Input: part model. Units: mm. Frame: model coordinates. Face numbers are marked on the shaded views. A direction names the side the tool comes from. Give positions to 0.01 mm unless a question says otherwise; leave off trailing zeros. Order: outer loops, then holes, each group sorted by start corner. A loop starts at its lowest first (then second) coordinate and runs counter-clockwise, first axis right, second up. Notation, with made-up numbers: M 50.5,-13 L 107.5,-13 A19 cw 107.5,8 Z; hole C 61.5,66 d2. An arc over 180 degrees is marked long. Use a Markdown table: item, result.
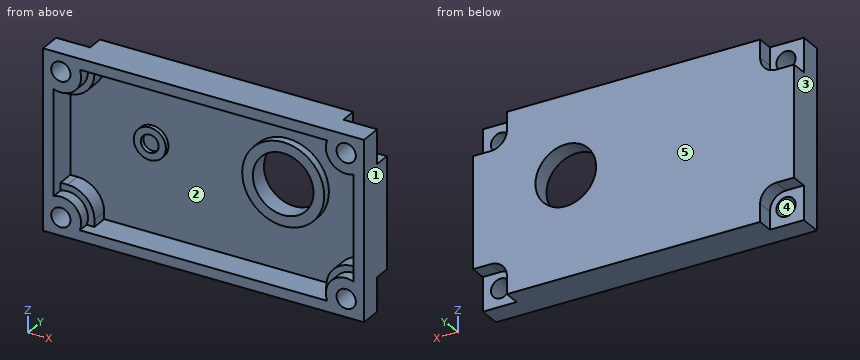
from build123d import *

# Parameters (mm, degrees)
SKETCH_1_W            = 45
SKETCH_1_H            = 25
EXTRUDE_1_DEPTH       = 5.4
SKETCH_2_R            = 1.35
CUT_EXTRUDE_1_DEPTH   = 27.299429652
CUT_EXTRUDE_2_DEPTH   = 2.3
MIRROR_2_COPY_1_DEPTH = 2.3
SHELL_1_DEPTH         = 3.9
SHELL_1_2_DEPTH       = 1.6
SKETCH_4_R            = 4.25
CUT_EXTRUDE_3_DEPTH   = 27.299429652
SKETCH_6_R            = 5.75
SKETCH_6_R_2          = 4.25
EXTRUDE_3_DEPTH       = 1.1
SKETCH_7_R            = 2.25
SKETCH_7_R_2          = 1.25
EXTRUDE_4_DEPTH       = 0.6


# Read off the part's stored shape, not the designer's step: 薄殼1
with BuildPart() as part:
    # 草圖1 → 填料-伸長1 (new body)
    with BuildSketch(Plane(origin=(0, 0, 0), x_dir=(1, 0, 0), z_dir=(0, 1, 0))):
        Rectangle(SKETCH_1_W, SKETCH_1_H)
    extrude(amount=EXTRUDE_1_DEPTH)

    # 草圖2 → 除料-伸長1 (cut, through all)
    with BuildSketch(Plane(origin=(0, 5.4, 0), x_dir=(1, 0, 0), z_dir=(0, 1, 0))):
        with Locations(Location((-20, 10, 0), (0, 0, 270))):
            Circle(SKETCH_2_R)
        with Locations(Location((-20, -10, 0), (0, 0, 270))):
            Circle(SKETCH_2_R)
        with Locations(Location((20, -10, 0), (0, 0, 270))):
            Circle(SKETCH_2_R)
        with Locations(Location((20, 10, 0), (0, 0, 270))):
            Circle(SKETCH_2_R)
    extrude(amount=-CUT_EXTRUDE_1_DEPTH, mode=Mode.SUBTRACT)

    # 草圖3 → 除料-伸長2 (cut)
    with BuildSketch(Plane(origin=(0, 5.4, 0), x_dir=(1, 0, 0), z_dir=(0, 1, 0))):
        with BuildLine():
            Line((-20, -7.75), (-22.5, -7.75))
            Line((-22.5, -7.75), (-22.5, -12.5))
            Line((-22.5, -12.5), (-17.75, -12.5))
            Line((-17.75, -12.5), (-17.75, -10))
            ThreePointArc((-17.75, -10), (-18.409009742, -8.409009742), (-20, -7.75))
        make_face()
    cut_extrude_2 = extrude(amount=-CUT_EXTRUDE_2_DEPTH, mode=Mode.SUBTRACT)

    # 鏡射1: 除料-伸長2 across plane
    add(cut_extrude_2.mirror(Plane.XY), mode=Mode.SUBTRACT)

    # 鏡射2: 除料-伸長2 across plane
    add(cut_extrude_2.mirror(Plane(origin=(0, 0, 0), x_dir=(0, 0, 1), z_dir=(1, 0, 0))), mode=Mode.SUBTRACT)

    # 鏡射2 copy 1 sketch → 鏡射2 copy 1 (cut)
    with BuildSketch(Plane(origin=(0, 5.4, 0), x_dir=(-1, 0, 0), z_dir=(0, 1, 0))):
        with BuildLine():
            Line((-20, -7.75), (-22.5, -7.75))
            Line((-22.5, -7.75), (-22.5, -12.5))
            Line((-22.5, -12.5), (-17.75, -12.5))
            Line((-17.75, -12.5), (-17.75, -10))
            ThreePointArc((-17.75, -10), (-18.409009742, -8.409009742), (-20, -7.75))
        make_face()
    extrude(amount=-MIRROR_2_COPY_1_DEPTH, mode=Mode.SUBTRACT)

    # 薄殼1 outline → 薄殼1 (cut)
    with BuildSketch(Plane(origin=(0, 0, 0), x_dir=(1, 0, 0), z_dir=(0, 1, 0))):
        with BuildLine():
            Line((-16.25, -11), (16.25, -11))
            Line((16.25, -11), (16.25, -10))
            ThreePointArc((16.25, -10), (17.348349571, -7.348349571), (20, -6.25))
            Line((20, -6.25), (21, -6.25))
            Line((21, -6.25), (21, 6.25))
            Line((21, 6.25), (20, 6.25))
            ThreePointArc((20, 6.25), (17.348349571, 7.348349571), (16.25, 10))
            Line((16.25, 10), (16.25, 11))
            Line((16.25, 11), (-16.25, 11))
            Line((-16.25, 11), (-16.25, 10))
            ThreePointArc((-16.25, 10), (-17.348349571, 7.348349571), (-20, 6.25))
            Line((-20, 6.25), (-21, 6.25))
            Line((-21, 6.25), (-21, -6.25))
            Line((-21, -6.25), (-20, -6.25))
            ThreePointArc((-20, -6.25), (-17.348349571, -7.348349571), (-16.25, -10))
            Line((-16.25, -10), (-16.25, -11))
        make_face()
    extrude(amount=SHELL_1_DEPTH, mode=Mode.SUBTRACT)

    # Shell 1 2 outline → Shell 1 2 (cut)
    with BuildSketch(Plane(origin=(0, 0, 0), x_dir=(1, 0, 0), z_dir=(0, 1, 0))):
        with BuildLine():
            Line((16.25, -11), (17.331198771, -11))
            ThreePointArc((17.331198771, -11), (17.984745674, -7.984745674), (21, -7.331198771))
            Line((21, -7.331198771), (21, -6.25))
            Line((21, -6.25), (20, -6.25))
            ThreePointArc((20, -6.25), (17.348349571, -7.348349571), (16.25, -10))
            Line((16.25, -10), (16.25, -11))
        make_face()
        with BuildLine():
            Line((-17.331198771, -11), (-16.25, -11))
            Line((-16.25, -11), (-16.25, -10))
            ThreePointArc((-16.25, -10), (-17.348349571, -7.348349571), (-20, -6.25))
            Line((-20, -6.25), (-21, -6.25))
            Line((-21, -6.25), (-21, -7.331198771))
            ThreePointArc((-21, -7.331198771), (-17.984745674, -7.984745674), (-17.331198771, -11))
        make_face()
        with BuildLine():
            Line((20, 6.25), (21, 6.25))
            Line((21, 6.25), (21, 7.331198771))
            ThreePointArc((21, 7.331198771), (17.984745674, 7.984745674), (17.331198771, 11))
            Line((17.331198771, 11), (16.25, 11))
            Line((16.25, 11), (16.25, 10))
            ThreePointArc((16.25, 10), (17.348349571, 7.348349571), (20, 6.25))
        make_face()
        with BuildLine():
            Line((-21, 7.331198771), (-21, 6.25))
            Line((-21, 6.25), (-20, 6.25))
            ThreePointArc((-20, 6.25), (-17.348349571, 7.348349571), (-16.25, 10))
            Line((-16.25, 10), (-16.25, 11))
            Line((-16.25, 11), (-17.331198771, 11))
            ThreePointArc((-17.331198771, 11), (-17.984745674, 7.984745674), (-21, 7.331198771))
        make_face()
    extrude(amount=SHELL_1_2_DEPTH, mode=Mode.SUBTRACT)

    # 草圖4 → 除料-伸長3 (cut, through all)
    with BuildSketch(Plane(origin=(0, 5.4, 0), x_dir=(1, 0, 0), z_dir=(0, 1, 0))):
        with Locations(Location((9.5, -1.5, 0), (0, 0, 270))):
            Circle(SKETCH_4_R)
    extrude(amount=-CUT_EXTRUDE_3_DEPTH, mode=Mode.SUBTRACT)

    # 草圖6 → 填料-伸長3 (add)
    with BuildSketch(Plane.XZ.offset(-3.9)):
        with Locations(Location((9.5, 1.5, 0), (0, 0, 90))):
            Circle(SKETCH_6_R)
        with Locations(Location((9.5, 1.5, 0), (0, 0, 90))):
            Circle(SKETCH_6_R_2, mode=Mode.SUBTRACT)
    extrude(amount=EXTRUDE_3_DEPTH)

    # 草圖7 → 填料-伸長4 (add)
    with BuildSketch(Plane.XZ.offset(-3.9)):
        with Locations(Location((-9.5, 1.5, 0), (0, 0, 90))):
            Circle(SKETCH_7_R)
        with Locations(Location((-9.5, 1.5, 0), (0, 0, 270))):
            Circle(SKETCH_7_R_2, mode=Mode.SUBTRACT)
    extrude(amount=EXTRUDE_4_DEPTH)


solid = part.part
1) Cut plane C-C on x = 9.5. Return loops of the section in (y, z).
Response values:
| item | result |
|---|---|
| outline | M 0,-12.5 L 5.4,-12.5 L 5.4,-2.75 L 2.8,-2.75 L 2.8,-4.25 L 3.9,-4.25 L 3.9,-11 L 0,-11 Z; M 0,11 L 3.9,11 L 3.9,7.25 L 2.8,7.25 L 2.8,5.75 L 5.4,5.75 L 5.4,12.5 L 0,12.5 Z |
2) Mould query, pull axis X, two halves, no side actions, for the marked faces 3, 4 and 5. Classes: released by +X, released by -X, zero draft, split by the parting line, or undercut.
Response values:
| item | result |
|---|---|
| face 3 | released by -X |
| face 4 | undercut |
| face 5 | zero draft |
3) Cut plane B-B on z = 1.5. Return loops of the section in (x, y).
Response values:
| item | result |
|---|---|
| outline | M -22.5,0 L -21,0 L -21,3.9 L -11.75,3.9 L -11.75,3.3 L -10.75,3.3 L -10.75,3.9 L -8.25,3.9 L -8.25,3.3 L -7.25,3.3 L -7.25,3.9 L 3.75,3.9 L 3.75,2.8 L 5.25,2.8 L 5.25,5.4 L -22.5,5.4 Z; M 13.75,2.8 L 15.25,2.8 L 15.25,3.9 L 21,3.9 L 21,0 L 22.5,0 L 22.5,5.4 L 13.75,5.4 Z |
4) Cut plane D-D on x = -4.5. Return loops of the section in (y, z).
Response values:
| item | result |
|---|---|
| outline | M 0,-12.5 L 5.4,-12.5 L 5.4,12.5 L 0,12.5 L 0,11 L 3.9,11 L 3.9,-11 L 0,-11 Z |
5) Material intervals for line 1 (Z direction, x = -14, y = 1.2); line 2 (Z direction, x = 5, y = 3.6); line 3 (X direction, y = 1.5, z = -10), sorted ascending. Write a range as from..to.
Response values:
| item | result |
|---|---|
| line 1 | z = -12.5..-11, 11..12.5 |
| line 2 | z = -12.5..-11, -2.08..5.08, 11..12.5 |
| line 3 | x = -22.5..-21.35, -18.65..-17.15, 17.15..18.65, 21.35..22.5 |
6) Cut plane A-A on y = 2.2. Return loops of the section in (x, z), and give its area (3 significant figures).
Response values:
| item | result |
|---|---|
| outline | M -22.5,-12.5 L 22.5,-12.5 L 22.5,12.5 L -22.5,12.5 Z; hole C -20,-10 d2.7; hole C -20,10 d2.7; hole M -21,-6.25 L -20,-6.25 A3.75 cw -16.25,-10 L -16.25,-11 L 16.25,-11 L 16.25,-10 A3.75 cw 20,-6.25 L 21,-6.25 L 21,6.25 L 20,6.25 A3.75 cw 16.25,10 L 16.25,11 L -16.25,11 L -16.25,10 A3.75 cw -20,6.25 L -21,6.25 Z; hole C 20,-10 d2.7; hole C 20,10 d2.7 |
| area | 256 mm² |
7) Reachability of the marked faces 1 and 2 from +Z, -Z, +X, -X, +Y, -Y: full face, straight path, thin tool, end or side. Return the list, or none.
Response values:
| item | result |
|---|---|
| face 1 | +Z, -Z, +X, +Y, -Y |
| face 2 | -Y |
8) First-contact query: pin 1 Ø1.5 at (x, z) = (2, -7.5) entering from -Y; pin 2 Ø2 at (x, z) = (-20, -10) entering from +Y; pin 3 Ø0.7 at (y, z) = (4.5, -11) entering from -X; pin 4 Ø2.5 at (x, z) = (-20.5, -11) entering from +Y. Flat tips, straight axial feed; report the tip coordinate or a pass-through.
Response values:
| item | result |
|---|---|
| pin 1 | stops at y = 3.9 |
| pin 2 | passes through |
| pin 3 | stops at x = -17.75 |
| pin 4 | stops at y = 3.1 |
